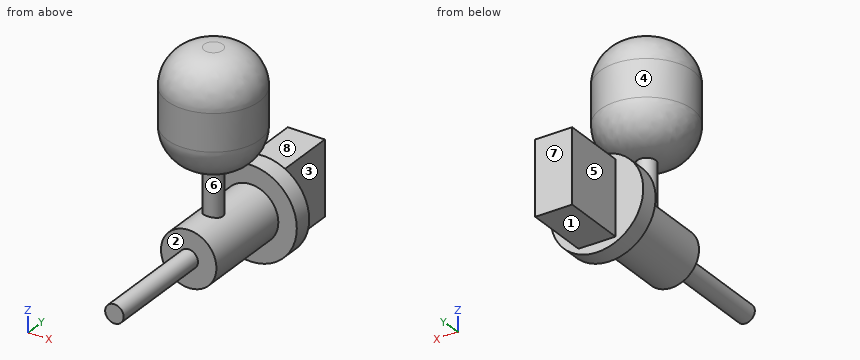
Autodesk Inventor part; units mm, degrees
ref_plane "YZ Plane" through (0, 0, 0) normal (1, 0, 0) x (0, 1, 0)
ref_plane "XZ Plane" through (0, 0, 0) normal (0, 1, 0) x (-1, 0, 0)
ref_plane "XY Plane" through (0, 0, 0) normal (0, 0, 1) x (1, 0, 0)
sketch "Skizze1" plane through (0, 0, 0) normal (0, 1, 0) x (-1, 0, 0)
  line L0 (10, -20) -> (-10, -20)
  line L1 (-10, -20) -> (-10, 20)
  line L2 (-10, 20) -> (10, 20)
  line L3 (10, 20) -> (10, -20)
  line L4 (10, -20) -> (-10, 20) construction
  line L5 (-10, -20) -> (10, 20) construction
  point P0 (0, 0)
  dimension "d0" = 20
  dimension "d1" = 40
extrude "Extrusion1" add sketch "Skizze1" along normal blind 35
sketch "Skizze2" plane through (0, 0, 0) normal (0, -1, 0) x (1, 0, 0)
  circle A0 centre (0, 0) radius 25
  dimension "d4" = 50
extrude "Extrusion2" add sketch "Skizze2" along normal blind 10
sketch "Skizze3" plane through (0, -10, 0) normal (0, -1, 0) x (1, 0, 0)
  circle A0 centre (0, 0) radius 15
  dimension "d7" = 30
extrude "Extrusion3" add sketch "Skizze3" along normal blind 50
sketch "Skizze4" plane through (0, 0, 0) normal (0, 0, 1) x (1, 0, 0)
  circle A0 centre (0, -40) radius 5
  point P0 (0, 0)
  dimension "d10" = 10
  dimension "d13" = 40
extrude "Extrusion4" add sketch "Skizze4" along normal blind 40
sketch "Skizze5" plane through (0, -40, 40) normal (0, 0, 1) x (1, 0, 0)
  circle A0 centre (0, 0) radius 25
  point P0 (0, 40)
  dimension "d14" = 50
extrude "Extrusion5" add sketch "Skizze5" along normal blind 60
fillet "Rundung1" radius 20 2 edges at (-25, -40, 100) (-25, -40, 40)
sketch "Skizze6" plane through (0, -60, 0) normal (0, -1, 0) x (1, 0, 0)
  circle A0 centre (0, 0) radius 5
  dimension "d18" = 10
extrude "Extrusion6" add sketch "Skizze6" along normal blind 60
properties part number "Lackierkopf"
Could you check a few things on this model? Use its own coordinates, in mm. Face numbers are marked on the shaded views. A direction names the side the tool comes from. Round coordinates to 2 decimals unless told otherwise and drop trailing zeros. Loops run counter-clockwise (first coordinate to the right, second up) from the corner with the lowest first, then second, coordinate; pieces in that order, holes last. Notation, with made-up numbers: (86.25, 49) - (95.25, 49) arc R28 ccw to (95.25, 80) - close; hole circle Ø3 at (2.5, 42). An arc over 180 degrees is marked (long way). Answer in a Markdown table with one row per item. Add a question column.
(1) If we section it at C-C (y = -96.5): Please give me the cut outline in (x, z), plus the area to 3 significant figures.
(2) I'm going to push flat-ended pins straight in: pin 1 (16 mm diameter, centred on x = -4.5, y = 24.5, fed in from -Z); pin 2 (2 mm diameter, centred on y = -17, z = 60, fed in from -X); pin 3 (11 mm diameter, centred on x = 0, y = -38.5, fed in from -Z). Where does each tip first touch, or does it pass through?
(3) I need wall thicknesses on line 1 along Z through (x, y) = (-5, 1); line 2 along X through (y, z) = (2.5, 12.5); line 3 along Z through (x, y) = (-6, -23). Which ranges of each line are inside material? Lowest first, please.
(4) If we section it at B-B (z = 23): Please give me the cut outline in (x, y), plus the area to 3 significant figures.
(5) For the marked faces 1, 2, 3, 4 and 5, which set-ups out of +Z, -Z, +X, -X, +Y, -Y let a thin tool reach every point of the face, with its end or its side?
(6) If we mould it in two halves opening along Z, with no side actions, what happens to the marked faces 6, 7 and 8? For each: pulls with the +Z half, pulls with the -Z half, needs draft (parallel to the pull), parting line crosses it, or undercut.
(7) If we section it at A-A (z = 0): Please give me the cut outline in (x, y), plus the area to 3 significant figures.
(8) If we section it at D-D (z = 72): Please give me the cut outline in (x, y), plus the area to 3 significant figures.
Model answer:
| question | item | result |
|---|---|---|
| 1 | outline | circle Ø10 at (0, 0) |
| 1 | area | 78.5 mm² |
| 2 | pin 1 | stops at z = -20 |
| 2 | pin 2 | stops at x = -11.87 |
| 2 | pin 3 | stops at z = -15 |
| 3 | line 1 | z = -20 to 20 |
| 3 | line 2 | x = -10 to 10 |
| 3 | line 3 | z = -13.75 to 13.75, 44.82 to 95.18 |
| 4 | outline | (-9.8, -10) - (9.8, -10) - (9.8, 0) - (-9.8, 0) - close; circle Ø10 at (0, -40) |
| 4 | area | 274 mm² |
| 5 | face 1 | -Z, +X, -X, +Y |
| 5 | face 2 | -Y |
| 5 | face 3 | +Z, -Z, +X, +Y |
| 5 | face 4 | +Z |
| 5 | face 5 | +Z, -Z, -X, +Y |
| 6 | face 6 | undercut |
| 6 | face 7 | needs draft |
| 6 | face 8 | pulls with the +Z half |
| 7 | outline | (-25, -10) - (-15, -10) - (-15, -60) - (-5, -60) - (-5, -120) - (5, -120) - (5, -60) - (15, -60) - (15, -10) - (25, -10) - (25, 0) - (10, 0) - (10, 35) - (-10, 35) - (-10, 0) - (-25, 0) - close |
| 7 | area | 3,300 mm² |
| 8 | outline | circle Ø50 at (0, -40) |
| 8 | area | 1,960 mm² |
